```python
from build123d import *

# Parameters (mm, degrees)
BOSS_EXTRUDE1_DEPTH      = 6
FILLET3_R                = 0.2
FILLET4_R                = 0.2
CIRPATTERN1_COUNT        = 10
FILLET3_OF_CIRPATTERN1_R = 0.2
FILLET4_OF_CIRPATTERN1_R = 0.2
CUT_EXTRUDE1_DEPTH       = 7
CUT_EXTRUDE1_DEPTH_BACK  = 6


with BuildPart() as part:
    # Sketch1 → Boss-Extrude1 (new body)
    with BuildSketch(Plane.XY):
        with BuildLine():
            Line((0, 0), (3.80266937, -1.235562177))
            ThreePointArc((3.80266937, -1.235562177), (3.87959472, -0.967291603), (3.937619073, -0.694308482))
            Line((3.937619073, -0.694308482), (4.579356052, -0.807464026))
            ThreePointArc((4.579356052, -0.807464026), (5.349965783, -0.745072725), (5.991777209, -0.314015737))
            ThreePointArc((5.991777209, -0.314015737), (6, 0), (5.991777209, 0.314015737))
            ThreePointArc((5.991777209, 0.314015737), (5.349965783, 0.745072725), (4.579356052, 0.807464026))
            Line((4.579356052, 0.807464026), (3.937619073, 0.694308482))
            ThreePointArc((3.937619073, 0.694308482), (3.87959472, 0.967291603), (3.80266937, 1.235562177))
            Line((3.80266937, 1.235562177), (0, 0))
        make_face()
    boss_extrude1 = extrude(amount=BOSS_EXTRUDE1_DEPTH)

    # Fillet3
    fillet3_edges = [part.edges().sort_by_distance(p)[0] for p in [
        (3.937619073, 0.694308482, 3),
    ]]
    fillet(fillet3_edges, radius=FILLET3_R)

    # Fillet4
    fillet4_edges = [part.edges().sort_by_distance(p)[0] for p in [
        (3.937619073, -0.694308482, 3),
    ]]
    fillet(fillet4_edges, radius=FILLET4_R)

    # CirPattern1: Boss-Extrude1 ×10 about axis
    cirpattern1_axis = Axis((0, 0, 0), (0, 0, 1))
    for i in range(1, CIRPATTERN1_COUNT):
        add(boss_extrude1.rotate(cirpattern1_axis, i * 360 / CIRPATTERN1_COUNT))

    # Fillet3 of CirPattern1
    fillet3_of_cirpattern1_edges = [part.edges().sort_by_distance(p)[0] for p in [
        (2.777496461, 2.876181782, 3),
        (0.556464605, 3.959451399, 3),
        (-1.877117817, 3.530345158, 3),
        (-3.593705034, 1.752767059, 3),
        (-3.937619073, -0.694308482, 3),
        (-2.777496461, -2.876181782, 3),
        (-0.556464605, -3.959451399, 3),
        (1.877117817, -3.530345158, 3),
        (3.593705034, -1.752767059, 3),
    ]]
    fillet(fillet3_of_cirpattern1_edges, radius=FILLET3_OF_CIRPATTERN1_R)

    # Fillet4 of CirPattern1
    fillet4_of_cirpattern1_edges = [part.edges().sort_by_distance(p)[0] for p in [
        (3.593705034, 1.752767059, 3),
        (1.877117817, 3.530345158, 3),
        (-0.556464605, 3.959451399, 3),
        (-2.777496461, 2.876181782, 3),
        (-3.937619073, 0.694308482, 3),
        (-3.593705034, -1.752767059, 3),
        (-1.877117817, -3.530345158, 3),
        (0.556464605, -3.959451399, 3),
        (2.777496461, -2.876181782, 3),
    ]]
    fillet(fillet4_of_cirpattern1_edges, radius=FILLET4_OF_CIRPATTERN1_R)

    # Sketch2 → Cut-Extrude1 (cut, two sides)
    with BuildSketch(Plane.XY) as cut_extrude1_sk:
        with BuildLine():
            Line((-0.988569227, 1.739), (-0.988569227, -1.739))
            ThreePointArc((-0.988569227, -1.739), (0, -2.000347499), (0.988569227, -1.739))
            Line((0.988569227, -1.739), (0.988569227, 1.739))
            ThreePointArc((0.988569227, 1.739), (0, 2.000347499), (-0.988569227, 1.739))
        make_face()
    extrude(amount=CUT_EXTRUDE1_DEPTH, mode=Mode.SUBTRACT)
    extrude(cut_extrude1_sk.sketch, amount=-CUT_EXTRUDE1_DEPTH_BACK, mode=Mode.SUBTRACT)


solid = part.part
```
The model under review builds one solid part; all positions refer to its coordinate system, in mm. A direction names the side the tool comes from. Coordinates: 2 decimals unless noted, no trailing zeros. Write each loop counter-clockwise with the first axis right and the second up, starting at its lowest first coordinate (ties: lowest second). Pieces come first, ordered by that corner, then holes.
1) To check wall thickness, follow probe 1 along X at (y, z) = (0.5, 3.9); probe 2 along Y at (x, z) = (-4, 2.65); probe 3 along X at (y, z) = (-1.5, 3.05). State the ranges of each line that lie inside material, in increasing order.
2) The part is to be moulded in two halves that separate along Y. For faces 1 (the face through (5.36, 0.74, 2.96)), 2 (the face through (0.951, 5.327, 2.958)), 3 (the face through (-3.9, -3.75, 2.96)), say which applies: pulls with the +Y half, pulls with the -Y half, needs draft (parallel to the pull), parting line crosses it, or undercut.
3) We need section A-A on y = 4.75. State the section outline as (x, z) points, then the cut area to 3 significant figures.
4) Machinability: for faces 4 (the face through (4.77, -2.55, 2.96)), 5 (the face through (-0.94, 5.31, 2.96)), 6 (the face through (-0.951, -5.327, 2.958)), 7 (the face through (-5.34, 0.75, 2.96)), which of the approach directions +Z, -Z, +X, -X, +Y, -Y give a long, thin tool a straight path to every point of the face, cutting with its end or side? Answer none if there is none.
5) We need section B-B on x = 5.25. State the section outline as (y, z) points.
6) Clearance check with flat-ended pins moving along their axes: pin 1 Ø1 at (x, z) = (4.5, 4.5) entering from +Y; pin 2 Ø1 at (x, z) = (1, 3) entering from +Y; pin 3 Ø3 at (y, z) = (-4.5, 3) entering from -X. State where each tip first meets the part, or that it passes through.
Answer list:
1. probe 1: x = -5.8 to -0.99, 0.99 to 5.8
1. probe 2: y = -3.78 to -1.95, -0.75 to 0.75, 1.95 to 3.78
1. probe 3: x = -3.71 to -0.99, 0.99 to 3.71
2. face 1: undercut
2. face 2: pulls with the +Y half
2. face 3: pulls with the -Y half
3. outline: (-2.36, 0) - (-0.67, 0) - (-0.67, 6) - (-2.36, 6) - close; (0.67, 0) - (2.36, 0) - (2.36, 6) - (0.67, 6) - close
3. area: 20.2 mm2
4. face 4: +Z, -Z, +X
4. face 5: +Z, -Z, +Y
4. face 6: +Z, -Z, -Y
4. face 7: +Z, -Z
5. outline: (-0.78, 0) - (0.78, 0) - (0.78, 6) - (-0.78, 6) - close
6. pin 1: stops at y = 3.81
6. pin 2: stops at y = 5.77
6. pin 3: stops at x = -5.03
